Build history of the part. All positions in model axes, mm. Give positions to 0.01 mm unless a question says otherwise; leave off trailing zeros. Loops run counter-clockwise (first coordinate to the right, second up) from the corner with the lowest first, then second, coordinate; pieces in that order, holes last.
1) Flat gauge pins, fed straight in: P1, Ø1.1, axis at x = -4, y = 5, coming from the +Z side; P2, Ø0.8, axis at x = -11.5, z = 3, coming from the +Y side. Where does each tip first touch, or does it go through?
2) Band-saw the part on C-C on x = 12.5. List the corners of the cut face in (y, z), then the cut area to 3 significant figures.
3) Band-saw the part on A-A on x = -6.35. List the corners of the cut face in (y, z).
4) Band-saw the part on D-D on x = 9. List the corners of the cut face in (y, z).
5) Wall check: line 1 (Y direction, x = -1, z = 3); line 2 (Y direction, x = 5.5, z = 0.25); line 3 (Z direction, x = 6, y = 5.5). Give the ranges that are in metal, low to high.
6) Band-saw the part on B-B on z = 0.75. List the corners of the cut face in (x, y).
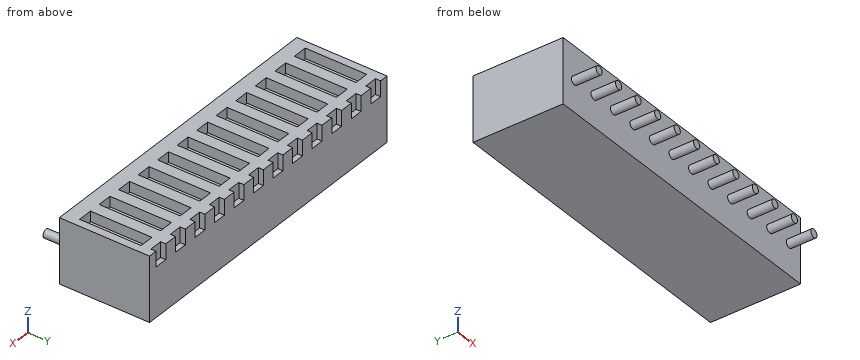
```python
from build123d import *

# Parameters (mm, degrees)
SKETCH2_W           = 30.88
SKETCH2_H           = 6.3
BOSS_EXTRUDE1_DEPTH = 8.8
SKETCH3_R           = 0.4
BOSS_EXTRUDE2_DEPTH = 2.4
SKETCH4_W           = 1.405361948
SKETCH4_H           = 6
CUT_EXTRUDE1_DEPTH  = 1
SKETCH5_W           = 1.27
SKETCH5_H           = 1.5
CUT_EXTRUDE2_DEPTH  = 0.5
LPATTERN1_COUNT     = 12
LPATTERN1_PITCH     = 2.54


with BuildPart() as part:
    # Sketch2 → Boss-Extrude1 (new body)
    with BuildSketch(Plane(origin=(0, 0, 0), x_dir=(1, 0, 0), z_dir=(0, 1, 0))):
        Rectangle(SKETCH2_W, SKETCH2_H)
    extrude(amount=BOSS_EXTRUDE1_DEPTH)

    # Sketch3 → Boss-Extrude2 (add)
    with BuildSketch(Plane.XZ):
        with Locations((-13.97, -0.15)):
            Circle(SKETCH3_R)
    boss_extrude2 = extrude(amount=BOSS_EXTRUDE2_DEPTH)

    # Sketch4 → Cut-Extrude1 (cut)
    with BuildSketch(Plane.XY.offset(3.15)):
        with Locations((-13.97, 4.4)):
            Rectangle(SKETCH4_W, SKETCH4_H)
    cut_extrude1 = extrude(amount=-CUT_EXTRUDE1_DEPTH, mode=Mode.SUBTRACT)

    # Sketch5 → Cut-Extrude2 (cut)
    with BuildSketch(Plane(origin=(0, 8.8, 0), x_dir=(1, 0, 0), z_dir=(0, 1, 0))):
        with Locations((-13.97, -2.4)):
            Rectangle(SKETCH5_W, SKETCH5_H)
    cut_extrude2 = extrude(amount=-CUT_EXTRUDE2_DEPTH, mode=Mode.SUBTRACT)

    # LPattern1: Boss-Extrude2, Cut-Extrude1, Cut-Extrude2 ×12
    with Locations(*[(i * LPATTERN1_PITCH, 0, 0) for i in range(1, LPATTERN1_COUNT)]):
        add(boss_extrude2)
        add(cut_extrude1, mode=Mode.SUBTRACT)
        add(cut_extrude2, mode=Mode.SUBTRACT)


solid = part.part
```
Findings below:
1. P1: stops at z = 3.15
1. P2: stops at y = 8.3
2. outline: (0, -3.15) - (8.8, -3.15) - (8.8, 3.15) - (0, 3.15) - close
2. area: 55.4 mm2
3. outline: (-2.4, -0.55) - (0, -0.55) - (0, -3.15) - (8.8, -3.15) - (8.8, 1.65) - (8.3, 1.65) - (8.3, 3.15) - (7.4, 3.15) - (7.4, 2.15) - (1.4, 2.15) - (1.4, 3.15) - (0, 3.15) - (0, 0.25) - (-2.4, 0.25) - close
4. outline: (-2.4, -0.53) - (0, -0.53) - (0, -3.15) - (8.8, -3.15) - (8.8, 1.65) - (8.3, 1.65) - (8.3, 3.15) - (7.4, 3.15) - (7.4, 2.15) - (1.4, 2.15) - (1.4, 3.15) - (0, 3.15) - (0, 0.23) - (-2.4, 0.23) - close
5. line 1: y = 0 to 1.4, 7.4 to 8.3
5. line 2: y = 0 to 8.8
5. line 3: z = -3.15 to 2.15
6. outline: (-15.44, 0) - (15.44, 0) - (15.44, 8.8) - (-15.44, 8.8) - close
